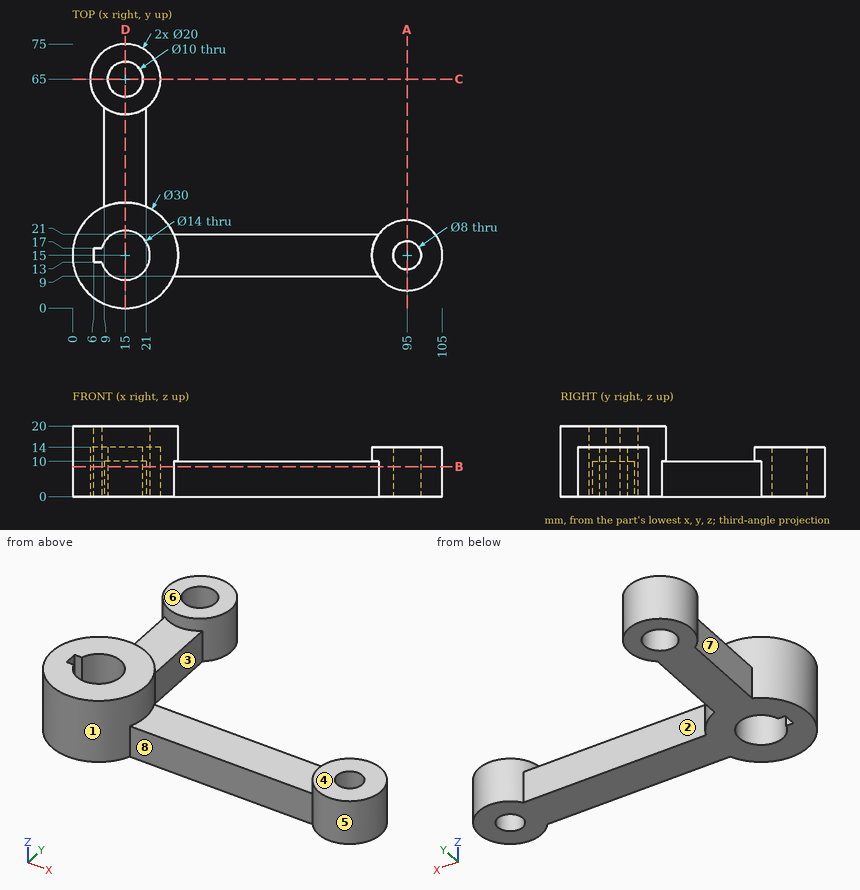
Input: dimensioned drawing with shaded views. Units: mm. Origin: part minimum x, y, z. A direction names the side the tool comes from. Give positions to 0.01 mm unless a question says otherwise; leave off trailing zeros. Write each loop counter-clockwise with the first axis right and the second up, starting at its lowest first coordinate (ties: lowest second). Pieces come first, ordered by that corner, then holes. Notation, with made-up numbers: (35, 27.25) - (62, 27.25) arc R13 ccw to (62, 32.25) - close; hole circle Ø2 at (37.25, 73.5). An arc over 180 degrees is marked (long way). Write item = value, one per line. Start each with the question number.
1) Cut plane D-D (x = 15). Return loops of the section in (y, z).
2) Reachability of the marked faces 1, 2, 3 and 4 from +Z, -Z, +X, -X, +Y, -Y: full face, straight path, thin tool, end or side. Return the list, or none.
3) Cut plane A-A (x = 95). Return loops of the section in (y, z).
4) Draft query along Y for the marked faces 5, 6, 7 and 8. Return one class per face: pulls with the +Y half, pulls with the -Y half, needs draft (parallel to the pull), parting line crosses it, or undercut.
5) Pin query (flat end, axial travel): pin 1 (3 mm diameter, centred on y = 39, z = 2.5, fed in from -X); pin 2 (11 mm diameter, centred on x = 59, z = 4.5, fed in from -Y); pin 3 (9.5 mm diameter, centred on x = 48.5, y = 16, fed in from +Z); pin 4 (22.5 mm diameter, centred on x = 15, y = 15, fed in from -Z). Return the tip coordinate at first contact, or that it passes through.
6) Cut plane B-B (z = 8.5). Return loops of the section in (x, y), and give its area (3 significant figures).
7) Material intervals for L1, parallel to X at y = 15, z = 9.5; L2, parallel to Y at x = 15, z = 11.25; L3, parallel to Y at x = 95, z = 5.25, sorted ascending. Write a range as [from, to].
8) Cut plane C-C (y = 65). Return loops of the section in (x, z).
Answers follow:
q1.outline = (0, 0) - (8, 0) - (8, 20) - (0, 20) - close; (22, 0) - (60, 0) - (60, 14) - (55, 14) - (55, 10) - (30, 10) - (30, 20) - (22, 20) - close; (70, 0) - (75, 0) - (75, 14) - (70, 14) - close
q2.face_1 = +Z
q2.face_2 = +Z, -Z, +Y
q2.face_3 = +Z, -Z, +X
q2.face_4 = +Z, +X, +Y, -Y
q3.outline = (5, 0) - (11, 0) - (11, 14) - (5, 14) - close; (19, 0) - (25, 0) - (25, 14) - (19, 14) - close
q4.face_5 = parting line crosses it
q4.face_6 = needs draft
q4.face_7 = undercut
q4.face_8 = pulls with the -Y half
q5.pin_1 = 9
q5.pin_2 = 9
q5.pin_3 = 10
q5.pin_4 = 0
q6.outline = (9, 28.75) arc R15 ccw (long way) to (28.75, 9) - (87, 9) arc R10 ccw (long way) to (87, 21) - (28.75, 21) arc R15 ccw to (21, 28.75) - (21, 57) arc R10 ccw (long way) to (9, 57) - close; hole (6, 13) - (8.29, 13) arc R7 ccw (long way) to (8.29, 17) - (6, 17) - close; hole circle Ø10 at (15, 65); hole circle Ø8 at (95, 15)
q6.area = 2,030 mm^2
q7.L1 = [0, 6], [22, 91], [99, 105]
q7.L2 = [0, 8], [22, 30], [55, 60], [70, 75]
q7.L3 = [5, 11], [19, 25]
q8.outline = (5, 0) - (10, 0) - (10, 14) - (5, 14) - close; (20, 0) - (25, 0) - (25, 14) - (20, 14) - close
